from build123d import *

# Parameters (mm, degrees)
SKETCH1_W           = 12.7
SKETCH1_H           = 1.5748
BOSS_EXTRUDE1_DEPTH = 3.048
SKETCH2_W           = 12.7
SKETCH2_H           = 0.1016
BOSS_EXTRUDE2_DEPTH = 3.048
SKETCH3_W           = 3.048
SKETCH3_H           = 7.2898
CUT_EXTRUDE1_DEPTH  = 4.048


with BuildPart() as part:
    # Sketch1 → Boss-Extrude1 (new body)
    with BuildSketch(Plane.XY):
        Polygon((-6.35, 1.5494), (-6.35, 4.7244), (3.048, 4.7244), (3.048, 9.8044), (0, 9.8044), (0, 16.1036), (3.048, 16.1036), (3.048, 21.1836), (0, 21.1836), (0, 24.0284), (-6.35, 24.0284), (-6.35, 27.2034), (-53.213, 27.2034), (-53.213, 24.0284), (-64.77, 24.0284), (-64.77, 27.2034), (-89.3064, 27.2034), (-89.3064, 15.9639), (-89.3064, 4.7244), (-86.7664, 4.7244), (-86.7664, 12.0142), (-84.963, 12.0142), (-84.963, 4.7244), (-46.863, 4.7244), (-46.863, 1.5494), align=None)
        with Locations((-78.613, 23.5458)):
            Rectangle(SKETCH1_W, SKETCH1_H, mode=Mode.SUBTRACT)
    extrude(amount=BOSS_EXTRUDE1_DEPTH)

    # Sketch2 → Boss-Extrude2 (add)
    with BuildSketch(Plane.XY.offset(3.048)):
        with Locations((-78.613, 24.384)):
            Rectangle(SKETCH2_W, SKETCH2_H)
    extrude(amount=-BOSS_EXTRUDE2_DEPTH)

    # Sketch3 → Cut-Extrude1 (cut, through all)
    with BuildSketch(Plane.XY.offset(3.048)):
        with Locations((-86.487, 8.3693)):
            Rectangle(SKETCH3_W, SKETCH3_H)
    extrude(amount=-CUT_EXTRUDE1_DEPTH, mode=Mode.SUBTRACT)


solid = part.part
The model under review builds one solid part; all positions refer to its coordinate system, in mm. A direction names the side the tool comes from. Give positions to 0.01 mm unless a question says otherwise; leave off trailing zeros. Order: outer loops, then holes, each group sorted by start corner. A loop starts at its lowest first (then second) coordinate and runs counter-clockwise, first axis right, second up. Notation, with made-up numbers: M -1.75,17 L 17.25,17 A15 cw 17.25,36 Z; hole C -5,-28 d1. An arc over 180 degrees is marked long. Use one line per item in the form item = value. Start each with the question number.
Item 1: We need section A-A on y = 8.75. Give the boundary of the cut face in (x, z), plus the area to 3 significant figures.
Item 2: To check wall thickness, follow line 1 along Y through (x, z) = (-75, 1.3); line 2 along X through (y, z) = (8.75, 1.65); line 3 along Y through (x, z) = (-48, 0.3). State the ranges of each line that lie inside material, in increasing order. Write a range as from..to.
Item 3: We need section D-D on x = -57.5. Give the boundary of the cut face in (y, z), plus the area to 3 significant figures.
Item 4: We need section B-B on x = -74. Give the boundary of the cut face in (y, z).
Item 5: We need section C-C on z = 0.65. Give the boundary of the cut face in (x, y), plus the area to 3 significant figures.
Item 6: The part is to be moulded in two halves that separate along X. For faces 1 (the flat face through (3.048, 7, 2)), 2 (the flat face through (-66, 4.724, 2)), 3 (the flat face through (-46.863, 3, 2)), 4 (the flat face through (-88.011, 8, 2)), say which applies: pulls with the +X half, pulls with the -X half, needs draft (parallel to the pull), parting line crosses it, or undercut.
Item 7: For faces 5 (the flat face through (-72.263, 24, 2)), 6 (the flat face through (-84.963, 8, 2)), 7 (the flat face through (-64.77, 26, 2)), 8 (the flat face through (2, 21.184, 2)), list the 3-axis set-ups (+Z, -Z, +X, -X, +Y, -Y) from which the entire face can be reached by the end or side of a thin tool; tool diameter is ignored.
Item 8: Insertion check: pin 1 Ø0.5 at (y, z) = (23.5, 1) entering from +X; pin 2 Ø1.5 at (x, z) = (-86, 1) entering from -Y; pin 3 Ø0.9 at (x, z) = (1.5, 1) entering from -Y. Each pin has a flat end and moves straight along its axis. Give the tip position at first contact, or say it passes through.
Completed:
q1.outline = M -89.31,0 L -88.01,0 L -88.01,3.05 L -89.31,3.05 Z; M -84.96,0 L 3.05,0 L 3.05,3.05 L -84.96,3.05 Z
q1.area = 272 mm²
q2.line_1 = 4.72..22.76, 24.33..27.2
q2.line_2 = -89.31..-88.01, -84.96..3.05
q2.line_3 = 4.72..27.2
q3.outline = M 4.72,0 L 24.03,0 L 24.03,3.05 L 4.72,3.05 Z
q3.area = 58.8 mm²
q4.outline = M 4.72,0 L 22.76,0 L 22.76,3.05 L 4.72,3.05 Z; M 24.33,0 L 27.2,0 L 27.2,3.05 L 24.33,3.05 Z
q5.outline = M -89.31,4.72 L -88.01,4.72 L -88.01,12.01 L -84.96,12.01 L -84.96,4.72 L -46.86,4.72 L -46.86,1.55 L -6.35,1.55 L -6.35,4.72 L 3.05,4.72 L 3.05,9.8 L 0,9.8 L 0,16.1 L 3.05,16.1 L 3.05,21.18 L 0,21.18 L 0,24.03 L -6.35,24.03 L -6.35,27.2 L -53.21,27.2 L -53.21,24.03 L -64.77,24.03 L -64.77,27.2 L -89.31,27.2 Z; hole M -84.96,22.76 L -72.26,22.76 L -72.26,24.33 L -84.96,24.33 Z
q5.area = 2,070 mm²
q6.face_1 = pulls with the +X half
q6.face_2 = needs draft
q6.face_3 = pulls with the -X half
q6.face_4 = undercut
q7.face_5 = +Z, -Z
q7.face_6 = +Z, -Z, -Y
q7.face_7 = +Z, -Z, +Y
q7.face_8 = +Z, -Z, +X, +Y
q8.pin_1 = 0
q8.pin_2 = 12.01
q8.pin_3 = 4.72
